Check sheet for the drawn part. Datum: minimum x, y, z corner. Units: mm. A direction names the side the tool comes from. Coordinates: 2 decimals unless noted, no trailing zeros. Loops run counter-clockwise (first coordinate to the right, second up) from the corner with the lowest first, then second, coordinate; pieces in that order, holes last.
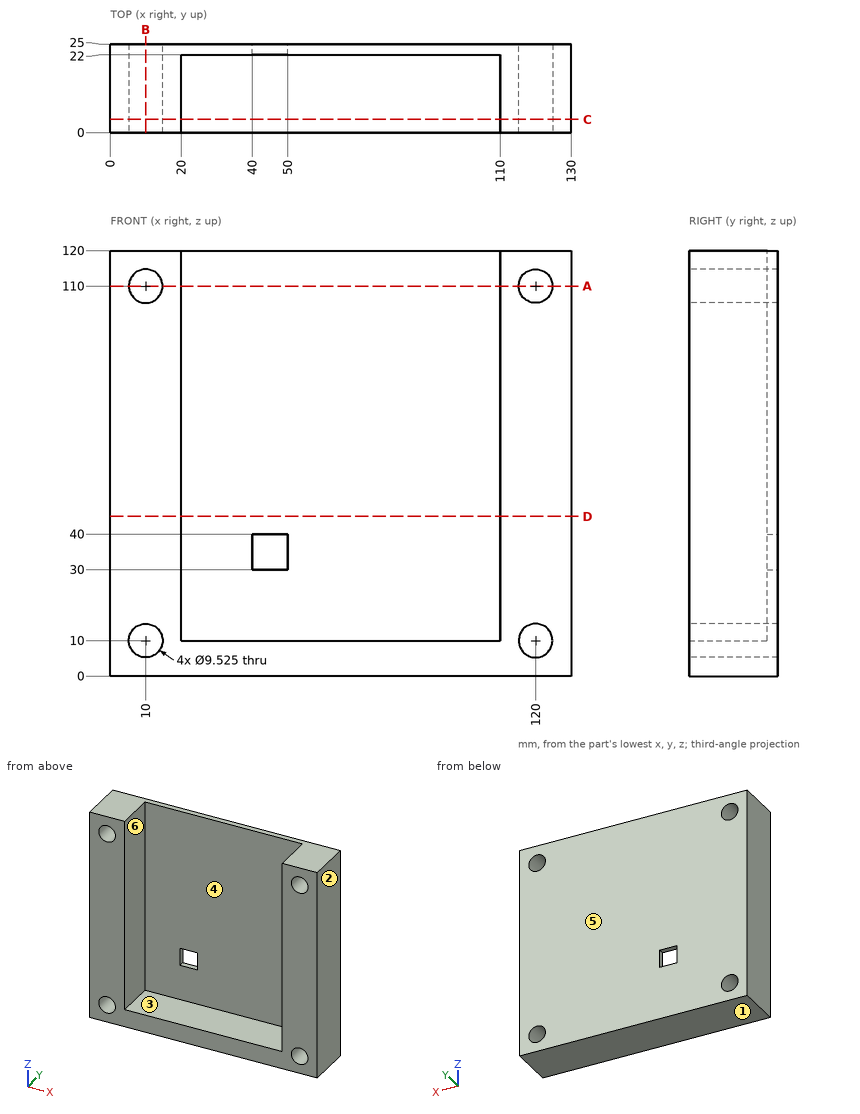
(1) Scan lines: L1, parallel to Z at x = 10, y = 13.5; L2, parallel to X at y = 15.5, z = 89.5; L3, parallel to X at y = 7.5, z = 107.5. Record each from-to range of solid material in increasing order.
Findings:
L1: z = 0 to 5.24, 14.76 to 105.24, 114.76 to 120
L2: x = 0 to 20, 110 to 130
L3: x = 0 to 5.95, 14.05 to 20, 110 to 115.95, 124.05 to 130
(2) Sectioned sample at A-A on z = 110. Record the cut outline in (x, y).
Findings:
outline: (0, 0) - (5.24, 0) - (5.24, 25) - (0, 25) - close; (14.76, 0) - (20, 0) - (20, 22) - (110, 22) - (110, 0) - (115.24, 0) - (115.24, 25) - (14.76, 25) - close; (124.76, 0) - (130, 0) - (130, 25) - (124.76, 25) - close
(3) Draft check along X on the marked faces 1, 2, 3 and 4. Enter one of: +X half, -X half, draft (parallel to the pull), parting line (faces both ways), or undercut.
Findings:
face 1: draft
face 2: +X half
face 3: undercut
face 4: undercut
(4) Access from +Z, -Z, +X, -X, +Y, -Y to the whole of each face (thin tool, end or side, straight path). Record for the marked faces 5 and 6.
Findings:
face 5: +Z, -Z, +X, -X, +Y
face 6: +Z, -Y
(5) Sectioned sample at C-C on y = 3.75. Record the cut outline in (x, z) (1 decimal), and give its area (3 significant figures).
Findings:
outline: (0, 0) - (130, 0) - (130, 120) - (110, 120) - (110, 10) - (20, 10) - (20, 120) - (0, 120) - close; hole circle Ø9.5 at (10, 10); hole circle Ø9.5 at (10, 110); hole circle Ø9.5 at (120, 10); hole circle Ø9.5 at (120, 110)
area: 5,410 mm2
(6) Gauge pin test, flat ends, axial feed: pin 1 Ø5.5 at (x, z) = (10, 10) entering from -Y; pin 2 Ø6.5 at (x, y) = (77, 16.5) entering from +Z; pin 3 Ø6 at (x, z) = (75, 56) entering from -Y. Record the tip position at first contact, or that the pin passes through.
Findings:
pin 1: passes through
pin 2: stops at z = 10
pin 3: stops at y = 22
(7) Sectioned sample at D-D on z = 45. Record the cut outline in (x, y), and give its area (3 significant figures).
Findings:
outline: (0, 0) - (20, 0) - (20, 22) - (110, 22) - (110, 0) - (130, 0) - (130, 25) - (0, 25) - close
area: 1,270 mm2
(8) Sectioned sample at B-B on x = 10. Record the cut outline in (y, z).
Findings:
outline: (0, 0) - (25, 0) - (25, 5.24) - (0, 5.24) - close; (0, 14.76) - (25, 14.76) - (25, 105.24) - (0, 105.24) - close; (0, 114.76) - (25, 114.76) - (25, 120) - (0, 120) - close
